```python
from build123d import *

# Parameters (mm, degrees)
SKETCH2_R               = 12.7
SKETCH2_R_2             = 11.1125
BOSS_EXTRUDE1_DEPTH     = 285.09415041
CUT_EXTRUDE1_DEPTH      = 286.659333119
CUT_EXTRUDE1_DEPTH_BACK = 286.659333119
SKETCH3_R               = 1.7526
CUT_EXTRUDE2_DEPTH      = 286.659333228
CUT_EXTRUDE2_DEPTH_BACK = 286.659333228
SKETCH4_R               = 1.7526


with BuildPart() as part:
    # Sketch2 → Boss-Extrude1 (new, symmetric)
    with BuildSketch(Plane.XY):
        Circle(SKETCH2_R)
        Circle(SKETCH2_R_2, mode=Mode.SUBTRACT)
    extrude(amount=BOSS_EXTRUDE1_DEPTH, both=True)

    # Sketch3 → Cut-Extrude1 (cut, two sides: drawn at the far end of the back side and taken through both)
    with BuildSketch(Plane(origin=(0, 0, 0), x_dir=(1, 0, 0), z_dir=(0, 1, 0)).offset(-CUT_EXTRUDE1_DEPTH_BACK)):
        with Locations(Location((0, -272.90215041, 0), (0, 0, 270))):
            Circle(SKETCH3_R)
        with Locations(Location((0, 272.90215041, 0), (0, 0, 270))):
            Circle(SKETCH3_R)
    extrude(amount=CUT_EXTRUDE1_DEPTH + CUT_EXTRUDE1_DEPTH_BACK, mode=Mode.SUBTRACT)

    # Sketch4 → Cut-Extrude2 (cut, two sides: drawn at the far end of the back side and taken through both)
    with BuildSketch(Plane(origin=(0, 0, 0), x_dir=(0, 0, -1), z_dir=(1, 0, 0)).offset(-CUT_EXTRUDE2_DEPTH_BACK)):
        with Locations((-272.90215041, 0)):
            Circle(SKETCH4_R)
        with Locations((272.90215041, 0)):
            Circle(SKETCH4_R)
    extrude(amount=CUT_EXTRUDE2_DEPTH + CUT_EXTRUDE2_DEPTH_BACK, mode=Mode.SUBTRACT)


solid = part.part
```
The model under review builds one solid part; all positions refer to its coordinate system, in mm. Round coordinates to 2 decimals unless told otherwise and drop trailing zeros. Order: outer loops, then holes, each group sorted by start corner. A loop starts at its lowest first (then second) coordinate and runs counter-clockwise, first axis right, second up. Notation, with made-up numbers: M 58,7.25 L 72,7.25 A37 cw 72,44.25 Z; hole C -37.75,56.25 d4. An arc over 180 degrees is marked long. Use a Markdown table: item, result.
1) Insertion check: pin 1 (5 mm diameter, centred on x = -4, z = -110.5, fed in from +Y); pin 2 (2 mm diameter, centred on x = -4, z = 141, fed in from -Y); pin 3 (2 mm diameter, centred on x = -7.5, z = -224, fed in from -Y). Each pin has a flat end and moves straight along its axis. Give the tip position at first contact, or say it passes through.
Report:
| item | result |
|---|---|
| pin 1 | y = 12.61 |
| pin 2 | y = -12.34 |
| pin 3 | y = -10.91 |
2) Wall thickness on line 1 along Z through (x, y) = (0, 12.1); line 2 along X through (y, z) = (-0.5, -150); line 3 along Y through (x, z) = (0.75, 234.5): over which ranges is each line inside the solid? List them lowest first. Write a range as [from, to].
Report:
| item | result |
|---|---|
| line 1 | [-285.09, -274.65], [-271.15, 271.15], [274.65, 285.09] |
| line 2 | [-12.69, -11.1], [11.1, 12.69] |
| line 3 | [-12.68, -11.09], [11.09, 12.68] |
3) Draft analysis for pull direction Y (two halves, no side actions). For faces 1 (the face through (-2.75, -12.4, 3.99)), 2 (the face through (10.6, 3.34, -3.99)), 3 (the face through (0.88, -11.23, 285.094)), state which applies: released by +Y, released by -Y, zero draft, split by the parting line, or undercut.
Report:
| item | result |
|---|---|
| face 1 | split by the parting line |
| face 2 | undercut |
| face 3 | zero draft |
4) Consider section B-B (z = -160.5). Write out the cut boundary in (x, y) (1 decimal), then the cut area to 3 significant figures.
Report:
| item | result |
|---|---|
| outline | C 0,0 d25.4; hole C 0,0 d22.2 |
| area | 119 mm^2 |
5) Consider section A-A (x = 6.25). Write out the cut boundary in (y, z).
Report:
| item | result |
|---|---|
| outline | M -11.06,-285.09 L -9.19,-285.09 L -9.19,285.09 L -11.06,285.09 Z; M 9.19,-285.09 L 11.06,-285.09 L 11.06,285.09 L 9.19,285.09 Z |
